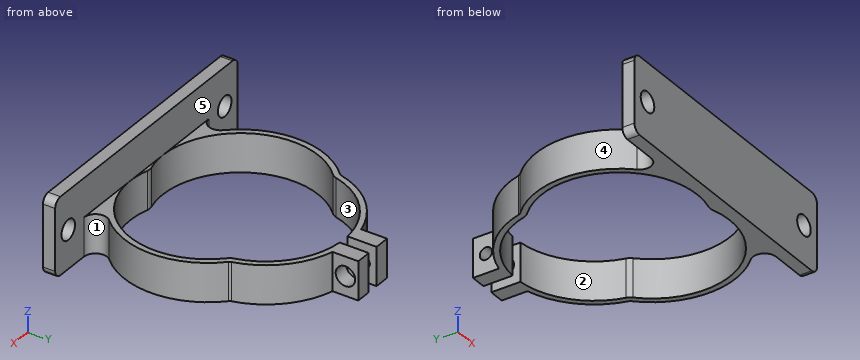
Autodesk Inventor part; units mm, degrees
ref_plane "YZ Plane" through (0, 0, 0) normal (1, 0, 0) x (0, 1, 0)
ref_plane "XZ Plane" through (0, 0, 0) normal (0, 1, 0) x (-1, 0, 0)
ref_plane "XY Plane" through (0, 0, 0) normal (0, 0, 1) x (1, 0, 0)
sketch "Block1" plane through (0, 0, 0) normal (0, 0, 1) x (1, 0, 0)
  arc A0 (0.8192, -22.866) -> (-0.8192, -22.866) centre (0, -25.7519) ccw construction
  arc A1 (-20.2121, 10.7235) -> (-19.3929, 12.1424) centre (-22.3018, 12.876) ccw construction
  circle A2 centre (21.4359, -12.376) radius 1.25 construction
  circle A3 centre (22.4424, 3.0852) radius 1.25 construction
  arc A4 (0.8192, -22.866) -> (20.2121, 10.7235) centre (6.2805, -3.626) ccw construction
  circle A5 centre (-8.5493, -20.9783) radius 1.25 construction
  circle A6 centre (8.5493, -20.9783) radius 1.25 construction
  circle A7 centre (-22.4424, 3.0852) radius 1.25 construction
  arc A8 (-20.2121, 10.7235) -> (-0.8192, -22.866) centre (-6.2805, -3.626) ccw construction
  circle A9 centre (-21.4359, -12.376) radius 1.25 construction
  arc A10 (19.3929, 12.1424) -> (20.2121, 10.7235) centre (22.3018, 12.876) ccw construction
  arc A11 (19.3929, 12.1424) -> (-19.3929, 12.1424) centre (0, 7.2521) ccw construction
  circle A12 centre (-13.8931, 17.8931) radius 1.25 construction
  circle A13 centre (13.8931, 17.8931) radius 1.25 construction
  circle A14 centre (0, 24.7521) radius 1.25 construction
  arc A15 (19.5868, 12.1913) -> (-19.5868, 12.1913) centre (0, 7.2521) ccw
  arc A16 (19.5868, 12.1913) -> (20.3514, 10.867) centre (22.3018, 12.876) ccw
  arc A17 (0.7646, -23.0584) -> (20.3514, 10.867) centre (6.2805, -3.626) ccw
  arc A18 (0.7646, -23.0584) -> (-0.7646, -23.0584) centre (0, -25.7519) ccw
  arc A19 (-20.3514, 10.867) -> (-0.7646, -23.0584) centre (-6.2805, -3.626) ccw
  arc A20 (-20.3514, 10.867) -> (-19.5868, 12.1913) centre (-22.3018, 12.876) ccw
  arc A21 (0.355, -24.5013) -> (-0.355, -24.5013) centre (0, -25.7519) ccw
  arc A22 (0.355, -24.5013) -> (21.3963, 11.9432) centre (6.2805, -3.626) ccw
  arc A23 (21.0413, 12.5581) -> (21.3963, 11.9432) centre (22.3018, 12.876) ccw
  arc A24 (21.0413, 12.5581) -> (-21.0413, 12.5581) centre (0, 7.2521) ccw
  arc A25 (-21.3963, 11.9432) -> (-21.0413, 12.5581) centre (-22.3018, 12.876) ccw
  arc A26 (-21.3963, 11.9432) -> (-0.355, -24.5013) centre (-6.2805, -3.626) ccw
  line L0 (-5.5, 28.2435) -> (-5.5, 34.9521)
  line L1 (-5.5, 34.9521) -> (-1.5, 34.9521)
  line L2 (-1.5, 34.9521) -> (-1.5, 27.3963)
  line L3 (0, 24.7521) -> (0, 36.4403) construction
  line L4 (5.5, 28.2435) -> (5.5, 34.9521)
  line L5 (5.5, 34.9521) -> (1.5, 34.9521)
  line L6 (1.5, 34.9521) -> (1.5, 27.3963)
  point P0 (0, 0)
  dimension "d0" = 0.2
  dimension "d1" = 1.5
  dimension "d2" = 1.5
  dimension "d3" = 4
  dimension "d4" = 6
sketch "Sketch2" plane through (0, 0, 0) normal (0, 0, 1) x (1, 0, 0)
  line L0 (-6.2805, -3.626) -> (0, 7.2521) construction
  line L1 (0, 7.2521) -> (6.2805, -3.626) construction
  line L2 (6.2805, -3.626) -> (-6.2805, -3.626) construction
  line L3 (-3.1402, 1.813) -> (0, 0) construction
  line L4 (0, 0) -> (3.1402, 1.813) construction
  line L5 (0, 0) -> (0, -3.626) construction
  arc A0 (0.8192, -22.866) -> (-0.8192, -22.866) centre (0, -25.7519) ccw construction
  arc A1 (-20.2121, 10.7235) -> (-19.3929, 12.1424) centre (-22.3018, 12.876) ccw construction
  circle A2 centre (21.4359, -12.376) radius 1.25 construction
  circle A3 centre (22.4424, 3.0852) radius 1.25 construction
  arc A4 (0.8192, -22.866) -> (20.2121, 10.7235) centre (6.2805, -3.626) ccw construction
  circle A5 centre (-8.5493, -20.9783) radius 1.25 construction
  circle A6 centre (8.5493, -20.9783) radius 1.25 construction
  circle A7 centre (-22.4424, 3.0852) radius 1.25 construction
  arc A8 (-20.2121, 10.7235) -> (-0.8192, -22.866) centre (-6.2805, -3.626) ccw construction
  circle A9 centre (-21.4359, -12.376) radius 1.25 construction
  arc A10 (19.3929, 12.1424) -> (20.2121, 10.7235) centre (22.3018, 12.876) ccw construction
  arc A11 (19.3929, 12.1424) -> (-19.3929, 12.1424) centre (0, 7.2521) ccw construction
  circle A12 centre (-13.8931, 17.8931) radius 1.25 construction
  circle A13 centre (13.8931, 17.8931) radius 1.25 construction
  circle A14 centre (0, 24.7521) radius 1.25 construction
  arc A15 (19.5868, 12.1913) -> (-19.5868, 12.1913) centre (0, 7.2521) ccw
  arc A16 (19.5868, 12.1913) -> (20.3514, 10.867) centre (22.3018, 12.876) ccw
  arc A17 (0.7646, -23.0584) -> (20.3514, 10.867) centre (6.2805, -3.626) ccw
  arc A18 (0.7646, -23.0584) -> (-0.7646, -23.0584) centre (0, -25.7519) ccw
  arc A19 (-20.3514, 10.867) -> (-0.7646, -23.0584) centre (-6.2805, -3.626) ccw
  arc A20 (-20.3514, 10.867) -> (-19.5868, 12.1913) centre (-22.3018, 12.876) ccw
  arc A21 (0.355, -24.5013) -> (-0.355, -24.5013) centre (0, -25.7519) ccw
  arc A22 (0.355, -24.5013) -> (21.3963, 11.9432) centre (6.2805, -3.626) ccw
  arc A23 (21.0413, 12.5581) -> (21.3963, 11.9432) centre (22.3018, 12.876) ccw
  arc A24 (21.0413, 12.5581) -> (-21.0413, 12.5581) centre (0, 7.2521) ccw
  arc A25 (-21.3963, 11.9432) -> (-21.0413, 12.5581) centre (-22.3018, 12.876) ccw
  arc A26 (-21.3963, 11.9432) -> (-0.355, -24.5013) centre (-6.2805, -3.626) ccw
  line L6 (-5.5, 28.2435) -> (-5.5, 34.9521)
  line L7 (-5.5, 34.9521) -> (-1.5, 34.9521)
  line L8 (-1.5, 34.9521) -> (-1.5, 27.3963)
  line L9 (0, 24.7521) -> (0, 36.4403) construction
  line L10 (5.5, 28.2435) -> (5.5, 34.9521)
  line L11 (5.5, 34.9521) -> (1.5, 34.9521)
  line L12 (1.5, 34.9521) -> (1.5, 27.3963)
extrude "Extrusion1" add sketch "Sketch2" along normal blind 10 contours A15 L12 A24 A23 A22 A21 A26 A25 L8 A20 A19 A18 A17 A16 | L12 L11 L10 A24 | A24 L6 L7 L8
sketch "Sketch3" plane through (5.5, 28.2435, 0) normal (1, 0, 0) x (0, 0, -1)
  line L0 (0, 6.7086) -> (-10, 6.7086) construction
  line L1 (-5, 6.7086) -> (-5, 0) construction
  line L2 (0, 0) -> (-10, 0) construction
  circle A0 centre (-5, 3.3543) radius 1.6
  point P0 (0, -28.2435)
  dimension "d7" = 3.2
extrude "Extrusion2" cut sketch "Sketch3" against normal through all
sketch "Sketch4" plane through (0, 0, 10) normal (0, 0, 1) x (1, 0, 0)
  line L0 (35, -27) -> (-35, -27)
  line L1 (-35, -27) -> (-35, -23.826)
  line L2 (-35, -23.826) -> (35, -23.826)
  line L3 (35, -23.826) -> (35, -27)
  arc A0 (-20.3514, 10.867) -> (-0.7646, -23.0584) centre (-6.2805, -3.626) ccw construction
  arc A1 (0.355, -24.5013) -> (-0.355, -24.5013) centre (0, -25.7519) ccw
  line L4 (0, -25.7519) -> (0, -23.826) construction
  point P0 (0, 0)
  dimension "d11" = 35
  dimension "d12" = 35
  dimension "d26" = 27
extrude "Extrusion3" add sketch "Sketch4" against normal up to surface (10 mm away)
fillet "Fillet1" radius 3 2 edges at (-14.2083, -23.826, 5) (14.2083, -23.826, 5)
sketch "Sketch6" plane through (0, 0, 10) normal (0, 0, 1) x (1, 0, 0)
  line L0 (-35, -27) -> (35, -27)
  line L1 (-35, -23.826) -> (-24.0076, -23.826)
  line L2 (35, -27) -> (-35, -27)
  line L3 (-35, -27) -> (-35, -23.826)
  line L4 (-35, -23.826) -> (35, -23.826)
  line L5 (35, -23.826) -> (35, -27)
  point P0 (0, 0)
extrude "Extrusion5" add sketch "Sketch6" along normal blind 10
sketch "Sketch5" plane through (35, -23.826, 10) normal (0, 1, 0) x (1, 0, 0)
  line L0 (0, 0) -> (-5, 0) construction
  circle A0 centre (-5, 0) radius 2.6
  line L1 (-70, 0) -> (-65, 0) construction
  circle A1 centre (-65, 0) radius 2.6
  line L2 (0, 10) -> (0, -10)
  line L3 (-70, -10) -> (-70, 10)
  point P0 (-35, 10)
  dimension "d16" = 5
  dimension "d17" = 5.2
extrude "Extrusion4" cut sketch "Sketch5" against normal blind 10
fillet "Fillet2" radius 2 4 edges at (35, -25.413, 0) (-35, -25.413, 0) (-35, -25.413, 20) (35, -25.413, 20)
sketch "Sketch7" plane through (5.5, 28.2435, 0) normal (1, 0, 0) x (0, 0, -1)
  circle A0 centre (-5, 3.3543) radius 1.6
  circle A1 centre (-5, 3.3543) radius 2.54
  point P0 (0, -28.2435)
  dimension "d23" = 5.08
extrude "Extrusion6" cut sketch "Sketch7" against normal up to surface (4 mm away) contours A0 | A1
equation "\"d12\" = d11"
properties part number "MotorTestBracket"
Design review of the part built by this model. Coordinates are the model's own, in mm. Face numbers are marked on the shaded views. A direction names the side the tool comes from. Coordinates: 2 decimals unless noted, no trailing zeros. Loops run counter-clockwise (first coordinate to the right, second up) from the corner with the lowest first, then second, coordinate; pieces in that order, holes last.
Q1. For pin 1 (8 mm diameter, centred on x = 23.5, y = -11, fed in from -Z); pin 2 (6 mm diameter, centred on x = -11.5, z = 13.5, fed in from +Y); pin 3 (8 mm diameter, centred on x = -13.5, y = 7.5, fed in from +Z); pin 4 (7.5 mm diameter, centred on y = 31, z = 2.5, fed in from -X), all flat-tipped, find the tip position at first contact; note any pin that passes through.
Reported:
pin 1: stops at z = 0
pin 2: stops at y = -23.83
pin 3: passes through
pin 4: stops at x = -8.42
Q2. We need section C-C on y = 15.5. State the section outline as (x, z) points.
Reported:
outline: (-20.07, 0) - (-18.44, 0) - (-18.44, 10) - (-20.07, 10) - close; (18.44, 0) - (20.07, 0) - (20.07, 10) - (18.44, 10) - close
Q3. We need section B-B on z = 9. State how many separate pieces and enclosed holes the cut face has, and give its area (3 significant figures).
Reported:
separate pieces: 3
enclosed holes: 0
area: 491 mm2
Q4. We need section D-D on x = 12.5. State the section outline as (y, z) points, and give its area (3 significant figures).
Reported:
outline: (-27, 0) - (-22.84, 0) - (-22.84, 10) - (-23.83, 10) - (-23.83, 20) - (-27, 20) - close; (23.12, 0) - (24.99, 0) - (24.99, 10) - (23.12, 10) - close
area: 92.0 mm2
Q5. To check wall thickness, follow line 1 (Z direction, x = 30, y = -24.8); line 2 (Y direction, x = -3.25, z = 5); line 3 (Y direction, x = 18, z = 13.5). State the ranges of each line that lie inside material, in increasing order.
Reported:
line 1: z = 0 to 7.4, 12.6 to 20
line 2: y = -27 to -23.6, 27.19 to 30, 33.2 to 34.95
line 3: y = -27 to -23.83
Q6. Tool access review of the marked faces 1 and 2: name each direction out of +Z, -Z, +X, -X, +Y, -Y from which nothing blocks a thin tool from reaching the whole face with its end or side.
Reported:
face 1: +Z, -Z, +X
face 2: +Z, -Z
Q7. We need section A-A on x = -30. State the section outline as (y, z) points.
Reported:
outline: (-27, 0) - (-23.83, 0) - (-23.83, 7.4) - (-27, 7.4) - close; (-27, 12.6) - (-23.83, 12.6) - (-23.83, 20) - (-27, 20) - close
Q8. The part is to be moulded in two halves that separate along X. For the marked faces 3, 4 and 5, say which applies: +X half, -X half, draft (parallel to the pull), parting line (faces both ways), or undercut.
Reported:
face 3: undercut
face 4: -X half
face 5: draft
